Source: CAD feature listing. Evaluate the final solid. Frame: model axes, mm. Face numbers are marked on the shaded views. A direction names the side the tool comes from. Coordinates: 2 decimals unless noted, no trailing zeros. Write each loop counter-clockwise with the first axis right and the second up, starting at its lowest first coordinate (ties: lowest second). Pieces come first, ordered by that corner, then holes. Notation, with made-up numbers: (29.5, 47) -> (41.5, 47) arc R31 cw to (41.5, 71) -> close; hole circle Ø6 at (-22.5, 15). An arc over 180 degrees is marked (long way). Write item = value, one per line.
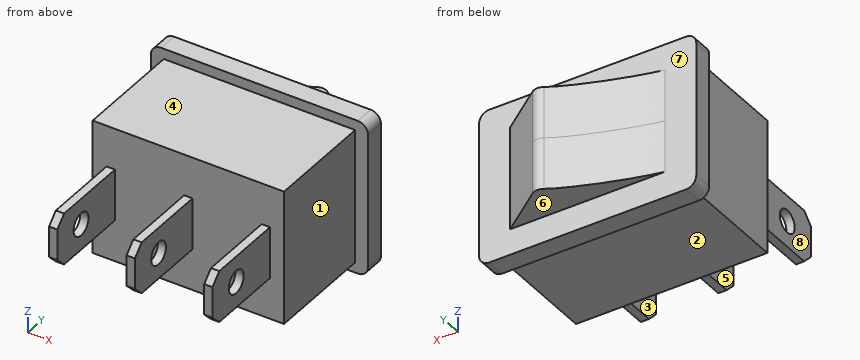
from build123d import *

# Parameters (mm, degrees)
SKETCH1_W           = 21
SKETCH1_H           = 15
BOSS_EXTRUDE1_DEPTH = 1.9
FILLET1_R           = 1
SKETCH2_W           = 18.5
SKETCH2_H           = 13
BOSS_EXTRUDE2_DEPTH = 10.5
BOSS_EXTRUDE3_START = -6.5
BOSS_EXTRUDE3_DEPTH = 5
FILLET2_R           = 1
SKETCH5_W           = 0.8
SKETCH5_H           = 5
BOSS_EXTRUDE4_DEPTH = 8.5
CHAMFER1_SIZE       = 1
SKETCH6_R           = 1.1
CUT_EXTRUDE1_DEPTH  = 28.491998836


with BuildPart() as part:
    # Sketch1 → Boss-Extrude1 (new body)
    with BuildSketch(Plane(origin=(0, 0, 0), x_dir=(1, 0, 0), z_dir=(0, 1, 0))):
        Rectangle(SKETCH1_W, SKETCH1_H)
    extrude(amount=BOSS_EXTRUDE1_DEPTH)

    # Fillet1
    fillet1_edges = [part.edges().sort_by_distance(p)[0] for p in [
        (10.5, 0.95, 7.5),
        (-10.5, 0.95, 7.5),
        (-10.5, 0.95, -7.5),
        (10.5, 0.95, -7.5),
    ]]
    fillet(fillet1_edges, radius=FILLET1_R)

    # Sketch2 → Boss-Extrude2 (add)
    with BuildSketch(Plane.XZ):
        Rectangle(SKETCH2_W, SKETCH2_H)
    extrude(amount=BOSS_EXTRUDE2_DEPTH)

    # Sketch4 → Boss-Extrude3 (add, symmetric)
    with BuildSketch(Plane(origin=(0, 0, -6.5), x_dir=(-1, 0, 0), z_dir=(0, 0, -1)).offset(BOSS_EXTRUDE3_START)):
        with BuildLine():
            Line((-7.5, 1.9), (7.5, 1.9))
            add(Edge.make_bspline(
                [(-2.5, 5.7), (-3.131503611, 3.8), (7.5, 1.9)],
                knots=[0, 0, 0, 2.456334169, 2.456334169, 2.456334169], degree=2, weights=[1, 0.335964667, 1]))
            Line((-2.5, 5.7), (-7.5, 1.9))
        make_face()
    extrude(amount=BOSS_EXTRUDE3_DEPTH, both=True)

    # Fillet2
    fillet2_edges = [part.edges().sort_by_distance(p)[0] for p in [
        (2.5, 5.7, -2.5),
    ]]
    fillet(fillet2_edges, radius=FILLET2_R)

    # Sketch5 → Boss-Extrude4 (add)
    with BuildSketch(Plane.XZ.offset(10.5)):
        with Locations((7.5, 0)):
            Rectangle(SKETCH5_W, SKETCH5_H)
        Rectangle(SKETCH5_W, SKETCH5_H)
        with Locations((-7.5, 0)):
            Rectangle(SKETCH5_W, SKETCH5_H)
    extrude(amount=BOSS_EXTRUDE4_DEPTH)

    # Chamfer1
    chamfer1_edges = [part.edges().sort_by_distance(p)[0] for p in [
        (0, -19, 2.5),
        (0, -19, -2.5),
        (7.5, -19, 2.5),
        (7.5, -19, -2.5),
        (-7.5, -19, 2.5),
        (-7.5, -19, -2.5),
    ]]
    chamfer(chamfer1_edges, length=CHAMFER1_SIZE)

    # Sketch6 → Cut-Extrude1 (cut, through all)
    with BuildSketch(Plane.ZY.offset(7.9)):
        with Locations((0, -15.5)):
            Circle(SKETCH6_R)
    extrude(amount=-CUT_EXTRUDE1_DEPTH, mode=Mode.SUBTRACT)


solid = part.part
1) Cut plane A-A, the plane y = -15.5. Output: boundary loops of the cut face in (x, z), and give its area (3 significant figures).
Answer block:
outline = (-7.9, -2.5) -> (-7.1, -2.5) -> (-7.1, -1.1) -> (-7.9, -1.1) -> close; (-7.9, 1.1) -> (-7.1, 1.1) -> (-7.1, 2.5) -> (-7.9, 2.5) -> close; (-0.4, -2.5) -> (0.4, -2.5) -> (0.4, -1.1) -> (-0.4, -1.1) -> close; (-0.4, 1.1) -> (0.4, 1.1) -> (0.4, 2.5) -> (-0.4, 2.5) -> close; (7.1, -2.5) -> (7.9, -2.5) -> (7.9, -1.1) -> (7.1, -1.1) -> close; (7.1, 1.1) -> (7.9, 1.1) -> (7.9, 2.5) -> (7.1, 2.5) -> close
area = 6.72 mm2
2) Reachability of the marked faces 4, 5, 6, 7 and 8 from +Z, -Z, +X, -X, +Y, -Y: full face, straight path, thin tool, end or side. Return the list, or none.
Answer block:
face_4 = +Z, +X, -X, -Y
face_5 = +Z, -Z, -Y
face_6 = -Z, +X, -X, +Y
face_7 = +Y
face_8 = +Z, -Z, -X, -Y
3) Cut plane B-B, the plane z = -5.5. Output: boundary loops of the cut face in (x, y).
Answer block:
outline = (-10.5, 0) -> (-9.25, 0) -> (-9.25, -10.5) -> (9.25, -10.5) -> (9.25, 0) -> (10.5, 0) -> (10.5, 1.9) -> (-10.5, 1.9) -> close
4) Material intervals for probe 1 along X at (y, z) = (-11, 0); probe 2 along Y at (x, z) = (-7.5, 0); probe 3 along Z at (x, y) = (1.75, -6.5), sorted ascending. Write a range as [from, to].
Answer block:
probe_1 = [-7.9, -7.1], [-0.4, 0.4], [7.1, 7.9]
probe_2 = [-19, -16.6], [-14.4, 1.9]
probe_3 = [-6.5, 6.5]
5) Pull-direction query (X, two-part tool) for the marked faces 1, 2 and 3; classes: +X half, -X half, draft (parallel to the pull), parting line (faces both ways), or undercut.
Answer block:
face_1 = +X half
face_2 = draft
face_3 = undercut
6) First-contact query: pin 1 Ø5 at (x, y) = (-4.5, -5) entering from +Z; pin 2 Ø1.5 at (y, z) = (-13.5, 0) entering from -X; pin 3 Ø2 at (x, z) = (-3, 1.5) entering from -Y. Flat tips, straight axial feed; report the tip coordinate or a pass-through.
Answer block:
pin_1 = 6.5
pin_2 = -7.9
pin_3 = -10.5
